from build123d import *

# Parameters (mm, degrees)
F0_R     = 2
F2_DEPTH = 5
F1_W     = 12
F1_H     = 11
F3_DEPTH = 50.9
F4_W     = 38
F4_H     = 15
F4_H_2   = 5
F5_DEPTH = 50
F6_DEPTH = 9
F7_W     = 16.1
F7_H     = 8
F8_DEPTH = 59.7
F9_DEPTH = 3.5


with BuildPart() as f2:
    # F0 (on Front) → F2 (new body)
    with BuildSketch(Plane.XZ):
        with BuildLine():
            ThreePointArc((-2.5, 0), (0, 2.5), (2.5, 0))
            Line((2.5, 0), (8, 0))
            Line((8, 0), (8, -3.5))
            Line((8, -3.5), (19, -3.5))
            Line((19, -3.5), (19, 12.5))
            Line((19, 12.5), (-19, 12.5))
            Line((-19, 12.5), (-19, 3.5))
            Line((-19, 3.5), (-8, 3.5))
            Line((-8, 3.5), (-8, 0))
            Line((-8, 0), (-2.5, 0))
        make_face()
        with Locations((13.25, 0)):
            Circle(F0_R, mode=Mode.SUBTRACT)
        with BuildLine():
            Line((8, 0), (2.5, 0))
            ThreePointArc((2.5, 0), (0, -2.5), (-2.5, 0))
            Line((-2.5, 0), (-8, 0))
            Line((-8, 0), (-8, 3.5))
            Line((-8, 3.5), (-19, 3.5))
            Line((-19, 3.5), (-19, -12.5))
            Line((-19, -12.5), (19, -12.5))
            Line((19, -12.5), (19, -3.5))
            Line((19, -3.5), (8, -3.5))
            Line((8, -3.5), (8, 0))
        make_face()
        with Locations((-13.25, 0)):
            Circle(F0_R, mode=Mode.SUBTRACT)
    extrude(amount=F2_DEPTH)

    # F1 (on Front) → F3 (cut)
    with BuildSketch(Plane.XZ):
        Rectangle(F1_W, F1_H)
    extrude(amount=F3_DEPTH, mode=Mode.SUBTRACT)

    # F4 (on face) → F5 (join)
    with BuildSketch(Plane.XY.offset(12.5)):
        with Locations((0, 7.5)):
            Rectangle(F4_W, F4_H)
        with Locations((0, -2.5)):
            Rectangle(F4_W, F4_H_2)
    extrude(amount=F5_DEPTH)

    # F6 (cut): a face of the model
    f6_faces = [f2.faces().sort_by_distance(p)[0] for p in [
        (0, 7.5, 12.5),
    ]]
    extrude(f6_faces, amount=-F6_DEPTH, mode=Mode.SUBTRACT)

    # F7 (on face) → F8 (cut)
    with BuildSketch(Plane.XY.offset(62.5)):
        with Locations((0, 4)):
            Rectangle(F7_W, F7_H)
    extrude(amount=-F8_DEPTH, mode=Mode.SUBTRACT)

    # F9 (cut): a face of the model
    f9_faces = [f2.faces().sort_by_distance(p)[0] for p in [
        (0, 15, 42),
    ]]
    extrude(f9_faces, amount=-F9_DEPTH, mode=Mode.SUBTRACT)


solid = f2.part
Can you work these out from the model? Positions are in its coordinate system, mm. A direction names the side the tool comes from. Coordinates: 2 decimals unless noted, no trailing zeros. Loops run counter-clockwise (first coordinate to the right, second up) from the corner with the lowest first, then second, coordinate; pieces in that order, holes last. Notation, with made-up numbers: (-16, 23) - (29, 23) arc R21 ccw to (29, 60) - close; hole circle Ø9 at (47.5, 3.25). An arc over 180 degrees is marked (long way). Answer as a JSON object with one key per item and string values. Group by question number.
Item 1: If we section it at A-A (y = 5.5): List the corners of the cut face in (x, z) for me.
Item 2: If we section it at D-D (x = -13.25): List the corners of the cut face in (y, z) for me.
Item 3: If we mould it in two halves opening along Z, with no side actions, what happens to faces 1 (the face through (0, -2, -12.5)), 2 (the face through (6, -2, 0)), 3 (the face through (-8.05, 4, 42))? For each: released by +Z, released by -Z, zero draft, split by the parting line, or undercut.
Item 4: On a 3-axis mill with a long thin cutter (end or side, diameter ignored), from which of +Z, -Z, +X, -X, +Y, -Y can I reach the whole of each face in a straight line? I mean faces 4 (the face through (-0.3, 8.4, 21.5)), 5 (the face through (0, 11.5, 42)), 6 (the face through (0, 0, 16)), 7 (the face through (0, 8, 42)), 8 (the face through (0, -2, 5.5)). Say none if no direction works.
Item 5: If we section it at B-B (x = 4): List the corners of the cut face in (y, z) for me, plus the area to 4 significant figures.
Item 6: If we section it at C-C (z = 0): List the corners of the cut face in (x, y) for me, plus the area to 3 significant figures.
Item 7: For pin 1 (3 mm diameter, centred on x = -12, y = 5, fed in from -Z), with a flat end and sliding along its axis, tell me the tip position at first contact or that it passes through.
Item 8: If I drill on L1, parallel to Z at x = -13.25, y = -2.3; L2, parallel to Z at x = 4.5, y = -4.5; L3, parallel to X at y = 4.5, z = 57.5, over which ranges is the centre line in solid material (lowest first)? Write a range as from..to.
Returned:
{
 "1": {"outline": "(-19, 21.5) - (-8.05, 21.5) - (-8.05, 62.5) - (-19, 62.5) - close; (8.05, 21.5) - (19, 21.5) - (19, 62.5) - (8.05, 62.5) - close"},
 "2": {"outline": "(-5, -12.5) - (0, -12.5) - (0, -2) - (-5, -2) - close; (-5, 2) - (0, 2) - (0, 21.5) - (11.5, 21.5) - (11.5, 62.5) - (-5, 62.5) - close"},
 "3": {"face 1": "released by -Z", "face 2": "undercut", "face 3": "zero draft"},
 "4": {"face 4": "-Z, +X, -X, +Y", "face 5": "+Z, -Z, +X, -X, +Y", "face 6": "-Z", "face 7": "+Z, -Z", "face 8": "+Y, -Y"},
 "5": {"outline": "(-5, -12.5) - (0, -12.5) - (0, -5.5) - (-5, -5.5) - close; (-5, 5.5) - (0, 5.5) - (0, 62.5) - (-5, 62.5) - close; (8, 21.5) - (11.5, 21.5) - (11.5, 62.5) - (8, 62.5) - close", "area": "463.5 mm²"},
 "6": {"outline": "(-19, -5) - (-15.25, -5) - (-15.25, 0) - (-19, 0) - close; (-11.25, -5) - (-6, -5) - (-6, 0) - (-11.25, 0) - close; (6, -5) - (11.25, -5) - (11.25, 0) - (6, 0) - close; (15.25, -5) - (19, -5) - (19, 0) - (15.25, 0) - close", "area": "90.0 mm²"},
 "7": {"pin 1": "stops at z = 21.5"},
 "8": {"L1": "z = -12.5..-2, 2..62.5", "L2": "z = -12.5..-5.5, 5.5..62.5", "L3": "x = -19..-8.05, 8.05..19"}
}
